Verification items for this drawing (mm, ordinates from the low corner). A direction names the side the tool comes from. Give positions to 0.01 mm unless a question says otherwise; leave off trailing zeros. Order: outer loops, then holes, each group sorted by start corner. A loop starts at its lowest first (then second) coordinate and runs counter-clockwise, first axis right, second up. Notation, with made-up numbers: M -23,-26.75 L 15,-26.75 A11 cw 15,-9.75 Z; hole C 51.25,-5.5 d2. An arc over 180 degrees is marked long. Answer as a JSON object with one key per item and string values.
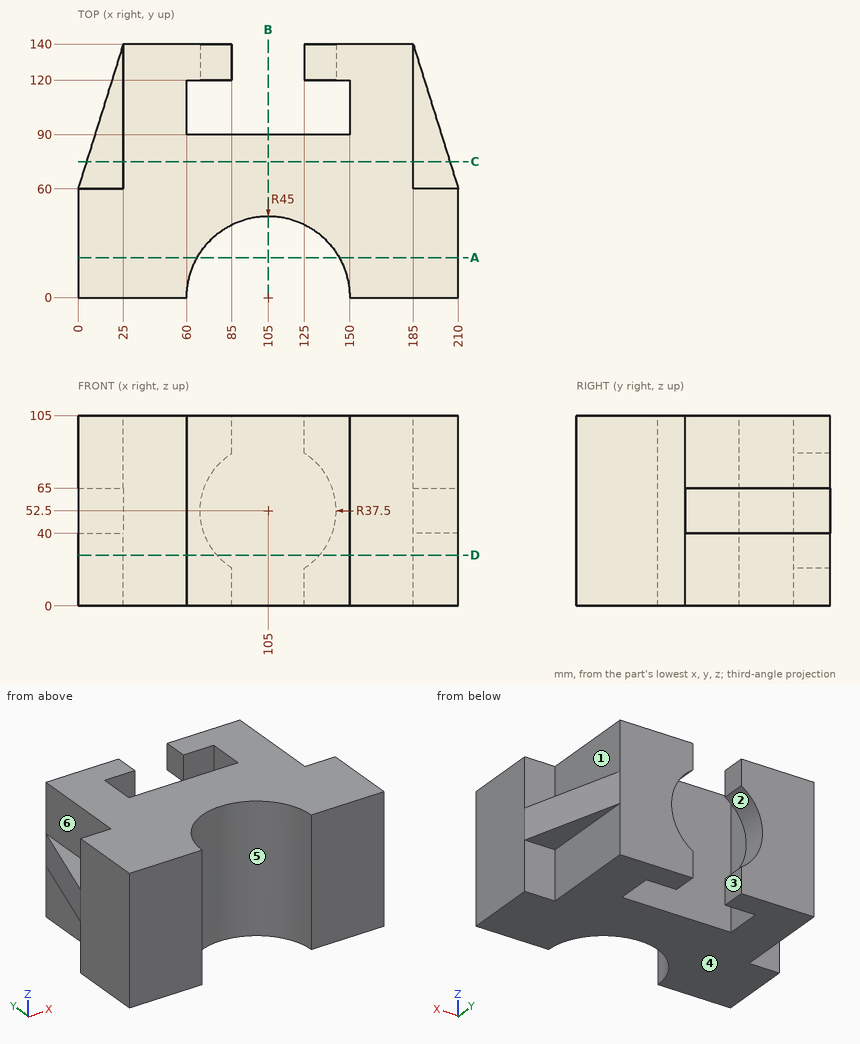
Q1. Section check A-A on y = 22. Record the cut outline in (x, z), then the cut area to 3 significant figures.
Resolved:
{"outline": "M 0,0 L 65.74,0 L 65.74,105 L 0,105 Z; M 144.26,0 L 210,0 L 210,105 L 144.26,105 Z", "area": "13,800 mm²"}
Q2. Section check C-C on y = 75. Record the cut outline in (x, z), then the cut area to 3 significant figures.
Resolved:
{"outline": "M 4.69,40 L 25,40 L 25,0 L 185,0 L 185,40 L 205.31,40 L 205.31,65 L 185,65 L 185,105 L 25,105 L 25,65 L 4.69,65 Z", "area": "17,800 mm²"}
Q3. Section check D-D on z = 28. Record the cut outline in (x, y).
Resolved:
{"outline": "M 0,0 L 60,0 A45 cw 150,0 L 210,0 L 210,60 L 185,60 L 185,140 L 133.39,140 L 133.39,120 L 150,120 L 150,90 L 60,90 L 60,120 L 76.61,120 L 76.61,140 L 25,140 L 25,60 L 0,60 Z"}
Q4. Section check B-B on x = 105. Record the cut outline in (y, z).
Resolved:
{"outline": "M 45,0 L 90,0 L 90,105 L 45,105 Z"}
Q5. Release check for a two-part mould opening along X. For the marked faces 4, 5 and 6 record: +X half, -X half, draft (parallel to the pull), parting line (faces both ways), or undercut.
Resolved:
{"face 4": "draft", "face 5": "undercut", "face 6": "-X half"}
Q6. Material ranges on L1, parallel to X at y = 107, z = 99; L2, parallel to X at y = 71, z = 29; L3, parallel to X at y = 100, z = 63, recorded low to high.
Resolved:
{"L1": "x = 25 to 60, 150 to 185", "L2": "x = 25 to 185", "L3": "x = 12.5 to 60, 150 to 197.5"}
Q7. Tool access check on the marked faces 1, 2 and 3. Record the directions out of +Z, -Z, +X, -X, +Y, -Y that give a thin tool (end or side, any length) a straight path to the whole face; none if there is none.
Resolved:
{"face 1": "+Z, +X, +Y", "face 2": "+Y", "face 3": "+Z, -Z, +Y"}
Q8. Gauge pin test, flat ends, axial feed: pin 1 Ø7.5 at (x, y) = (14.5, 105.5) entering from +Z; pin 2 Ø10 at (y, z) = (133.5, 10.5) entering from -X; pin 3 Ø22 at (y, z) = (129.5, 90.5) entering from +X; pin 4 Ø12.5 at (x, y) = (203, 104.5) entering from +Z (3 decimals). Record the tip position at first contact, or that the pin passes through.
Resolved:
{"pin 1": "stops at z = 65", "pin 2": "stops at x = 25", "pin 3": "stops at x = 185", "pin 4": "passes through"}
